Part model, mm, in its own coordinate system. Face numbers are marked on the shaded views. A direction names the side the tool comes from. Give positions to 0.01 mm unless a question says otherwise; leave off trailing zeros. Order: outer loops, then holes, each group sorted by start corner. A loop starts at its lowest first (then second) coordinate and runs counter-clockwise, first axis right, second up. Notation, with made-up numbers: M -28.75,22.25 L 0.25,22.25 A14 cw 0.25,27.25 Z; hole C 39.25,-12.5 d4. An arc over 180 degrees is marked long. Return JSON: item names as keys, results as strings.
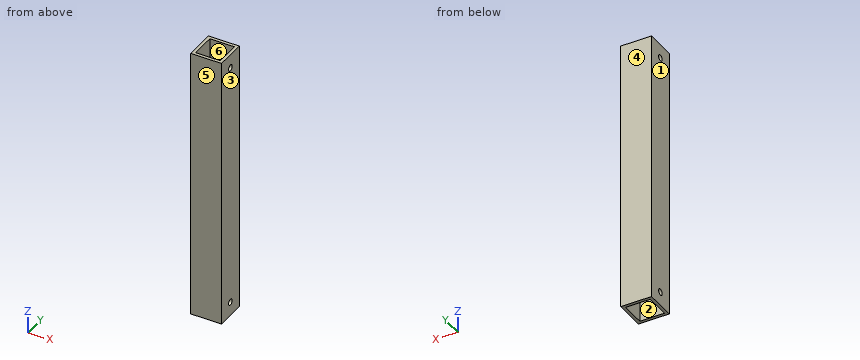
from build123d import *

# Parameters (mm, degrees)
SKETCH_1_W          = 20
SKETCH_1_H          = 20
SKETCH_1_W_2        = 16
SKETCH_1_H_2        = 16
EXTRUDE_1_DEPTH     = 90
SKETCH_2_R          = 2
CUT_EXTRUDE_1_DEPTH = 93.736184955
CUT_EXTRUDE_2_DEPTH = 93.736184955


with BuildPart() as part:
    # 草图1 → 凸台-拉伸1 (new, symmetric)
    with BuildSketch(Plane.XY):
        Rectangle(SKETCH_1_W, SKETCH_1_H)
        Rectangle(SKETCH_1_W_2, SKETCH_1_H_2, mode=Mode.SUBTRACT)
    extrude(amount=EXTRUDE_1_DEPTH, both=True)

    # 草图2 → 切除-拉伸1 (cut, through all)
    with BuildSketch(Plane(origin=(10, 0, 0), x_dir=(0, 0, -1), z_dir=(1, 0, 0))):
        with Locations(Location((80, 0, 0), (0, 0, 90))):
            Circle(SKETCH_2_R)
        with Locations(Location((-80, 0, 0), (0, 0, 90))):
            Circle(SKETCH_2_R)
    extrude(amount=-CUT_EXTRUDE_1_DEPTH, mode=Mode.SUBTRACT)

    # 草图3 → 切除-拉伸2 (cut, through all)
    with BuildSketch(Plane(origin=(10, 0, 0), x_dir=(0, 0, -1), z_dir=(1, 0, 0))):
        Polygon((-90, 10), (-89, 10), (-89, -15.299098046), (-95.501418201, -15.299098046), (-95.501418201, 10), align=None)
        Polygon((89, -15.299098046), (95.501418201, -15.299098046), (95.501418201, 10), (90, 10), (89, 10), align=None)
    extrude(amount=-CUT_EXTRUDE_2_DEPTH, mode=Mode.SUBTRACT)


solid = part.part
Q1. 3-axis set-ups, long thin cutter, end or side, ignore diameter. For the marked faces 5 and 6: which of +Z, -Z, +X, -X, +Y, -Y reach the whole face in a straight line?
Established:
{"face 5": "+Z, -Z, +X, -X, -Y", "face 6": "+Z, -Z"}
Q2. Band-saw the part on D-D (z = 0). Give the cut face in (x, y).
Established:
{"outline": "M -10,-10 L 10,-10 L 10,10 L -10,10 Z; hole M -8,-8 L 8,-8 L 8,8 L -8,8 Z"}
Q3. Band-saw the part on C-C (z = 80). Give the cut face in (x, y).
Established:
{"outline": "M -10,-10 L 10,-10 L 10,-2 L 8,-2 L 8,-8 L -8,-8 L -8,-2 L -10,-2 Z; M -10,2 L -8,2 L -8,8 L 8,8 L 8,2 L 10,2 L 10,10 L -10,10 Z"}
Q4. Pin check, flat tip, straight feed: pin 1 (2.5 mm diameter, centred on y = 0, z = 80, fed in from +X). Stop position of the tip, or through.
Established:
{"pin 1": "passes through"}
Q5. Band-saw the part on A-A (y = -4.75). Give the cut face in (x, z).
Established:
{"outline": "M -10,-89 L -8,-89 L -8,89 L -10,89 Z; M 8,-89 L 10,-89 L 10,89 L 8,89 Z"}
Q6. Probe line 1 along Z through (x, y) = (8.45, 0); line 2 along X through (y, z) = (7.5, 65.5). List the from-to ranges inside material, lowest first.
Established:
{"line 1": "z = -89 to -82, -78 to 78, 82 to 89", "line 2": "x = -10 to -8, 8 to 10"}
Q7. Two-plate mould, pull along X, no slides. Class the marked faces 1, 2, 3 and 4: +X half, -X half, draft (parallel to the pull), parting line (faces both ways), or undercut.
Established:
{"face 1": "-X half", "face 2": "undercut", "face 3": "+X half", "face 4": "draft"}
